Part model, mm, in its own coordinate system. Round coordinates to 2 decimals unless told otherwise and drop trailing zeros. Use CSV: the item, a comma, the result in double quotes.
Autodesk Inventor part; units mm, degrees
ref_plane "Work Plane1" through (7.5, 10, 710) normal (1, 0, 0) x (0, 0, -1)
ref_plane "YZ Plane" through (0, 0, 0) normal (1, 0, 0) x (0, 1, 0)
ref_plane "XZ Plane" through (0, 0, 0) normal (0, 1, 0) x (-1, 0, 0)
sketch "Sketch1" plane through (0, 0, 0) normal (0, 0, 1) x (1, 0, 0)
  line L0 (0, 0) -> (15, 0)
  line L1 (15, 0) -> (15, 10)
  line L2 (15, 10) -> (0, 10)
  line L3 (0, 10) -> (0, 0)
  dimension "d0" = 15
  dimension "d1" = 10
extrude "Extrusion1" add sketch "Sketch1" along normal blind 710
ref_plane "Work Plane1" through (7.5, 10, 710) normal (1, 0, 0) x (0, 0, -1)
sketch "Sketch4" plane through (7.5, 10, 710) normal (1, 0, 0) x (0, 0, -1)
  line L0 (692, 0) -> (692, -4.5)
  line L1 (698, -4.5) -> (698, 0)
  line L2 (692, -4.5) -> (693.25, -4.5)
  line L3 (693.25, -4.5) -> (693.25, -10)
  line L4 (693.25, -10) -> (696.75, -10)
  line L5 (696.75, -10) -> (696.75, -4.5)
  line L6 (696.75, -4.5) -> (698, -4.5)
  line L7 (710, 0) -> (0, 0)
  line L8 (710, -10) -> (0, -10)
  line L9 (692, 0) -> (698, 0)
  line L10 (695, -10) -> (695, 0)
  point P0 (698, -2.25)
  point P1 (695, 0)
  dimension "d6" = 6
  dimension "d7" = 3.5
  dimension "d8" = 4.5
  dimension "d9" = 15
revolve "Revolution1" cut sketch "Sketch4" angle 360 about axis through (7.5, 0, 15) along (0, -1, 0) contours L7 L1 L6 L5 L4 L10
pattern_linear "Rectangular Pattern1" count 20 spacing 40 along (0, 0, 1) of "Revolution1"
properties part number "MGN15H-750"
(1) Drop a flat-ended pin along its axis: P1, Ø1.8, axis at x = 7, z = 536.5, coming from the +Y side. Give the stop position or say it passes through.
Reply:
P1,"y = 5.5"
(2) Probe probe 1 along X at (y, z) = (3.2, 615); probe 2 along X at (y, z) = (7.6, 255); probe 3 along Y at (x, z) = (8.5, 413.5). List the from-to ranges inside material, lowest first. Write a range as [from, to].
Reply:
probe 1,"[0, 5.75], [9.25, 15]"
probe 2,"[0, 4.5], [10.5, 15]"
probe 3,"[0, 5.5]"
(3) Cut at A-A, the plane y = 3. State how many separate pieces and enclosed holes the cut face has, then the cut area to 3 significant figures.
Reply:
separate pieces,"1"
enclosed holes,"18"
area,"10,500 mm2"
